from build123d import *

# Parameters (mm, degrees)
F0_R     = 10.4775
F1_DEPTH = 76.2
F2_SIZE2 = 8.7988181024
F2_SIZE  = 5.08
F3_R     = 6.8453
F4_DEPTH = 76.201


with BuildPart() as f1:
    # F0 (on Top) → F1 (new body)
    with BuildSketch(Plane.XY):
        Circle(F0_R)
    extrude(amount=F1_DEPTH)

    # F2
    f2_edges = [f1.edges().sort_by_distance(p)[0] for p in [
        (-10.4775, 0, 76.2),
    ]]
    f2_side = f1.faces().sort_by_distance((0, 0, 76.2))[0]
    chamfer(f2_edges, length=F2_SIZE, length2=F2_SIZE2, reference=f2_side)

    # F3 (on face) → F4 (cut, through all)
    with BuildSketch(Plane(origin=(0, 0, 0), x_dir=(1, 0, 0), z_dir=(0, 0, -1))):
        Circle(F3_R)
    extrude(amount=-F4_DEPTH, mode=Mode.SUBTRACT)


solid = f1.part
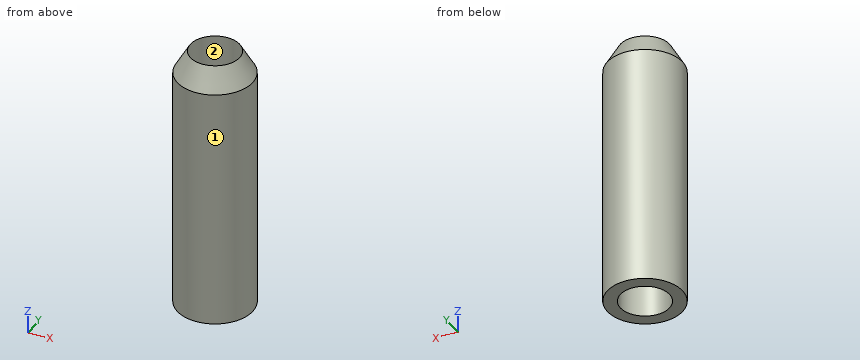
Source: CAD feature listing. Evaluate the final solid. Frame: model axes, mm. Face numbers are marked on the shaded views. Coordinates: 2 decimals unless noted, no trailing zeros. Loops run counter-clockwise (first coordinate to the right, second up) from the corner with the lowest first, then second, coordinate; pieces in that order, holes last. Notation, with made-up numbers: (15.5, 67.25) - (39.5, 67.25) arc R18 ccw to (39.5, 102.25) - close; hole circle Ø9 at (70.5, -24.5). An arc over 180 degrees is marked (long way). One line per item, written item: value. Start each with the question number.
1. Mould query, pull axis Y, two halves, no side actions, for the marked faces 1 and 2. Classes: pulls with the +Y half, pulls with the -Y half, needs draft (parallel to the pull), parting line crosses it, or undercut.
2. Section A-A (x = 0). Return the cut outline in (y, z).
3. Ray query, L1, parallel to Y at x = 0, z = 43; L2, parallel to X at y = -5.5, z = 40.5; L3, parallel to Y at x = 1.25, z = 31.5. Return the intervals inside material, ascending.
4. Contact query for flat-ended pins moving along their axis: P1, Ø1, axis at y = 7.5, z = 62.5, coming from the -X side; P2, Ø1.5, axis at x = -1.5, y = 6.5, coming from the +Z side; P3, Ø1, axis at y = -2.5, z = 26, coming from the -X side; P4, Ø1, axis at x = 5, y = 2.5, coming from the -Z side. Output: stop coordinate, or through.
5. Section C-C (z = 9). Return the cut outline in (x, y) (1 decimal), and give its area (3 significant figures).
Verdict:
1. face 1: parting line crosses it
1. face 2: undercut
2. outline: (-10.48, 0) - (-6.85, 0) - (-6.85, 73.69) - (-10.48, 67.4) - close; (6.85, 0) - (10.48, 0) - (10.48, 67.4) - (6.85, 73.69) - close
3. L1: y = -10.48 to -6.85, 6.85 to 10.48
3. L2: x = -8.92 to -4.08, 4.08 to 8.92
3. L3: y = -10.4 to -6.73, 6.73 to 10.4
4. P1: stops at x = -7.8
4. P2: stops at z = 73.69
4. P3: stops at x = -10.28
4. P4: passes through
5. outline: circle Ø21 at (0, 0); hole circle Ø13.7 at (0, 0)
5. area: 198 mm2
